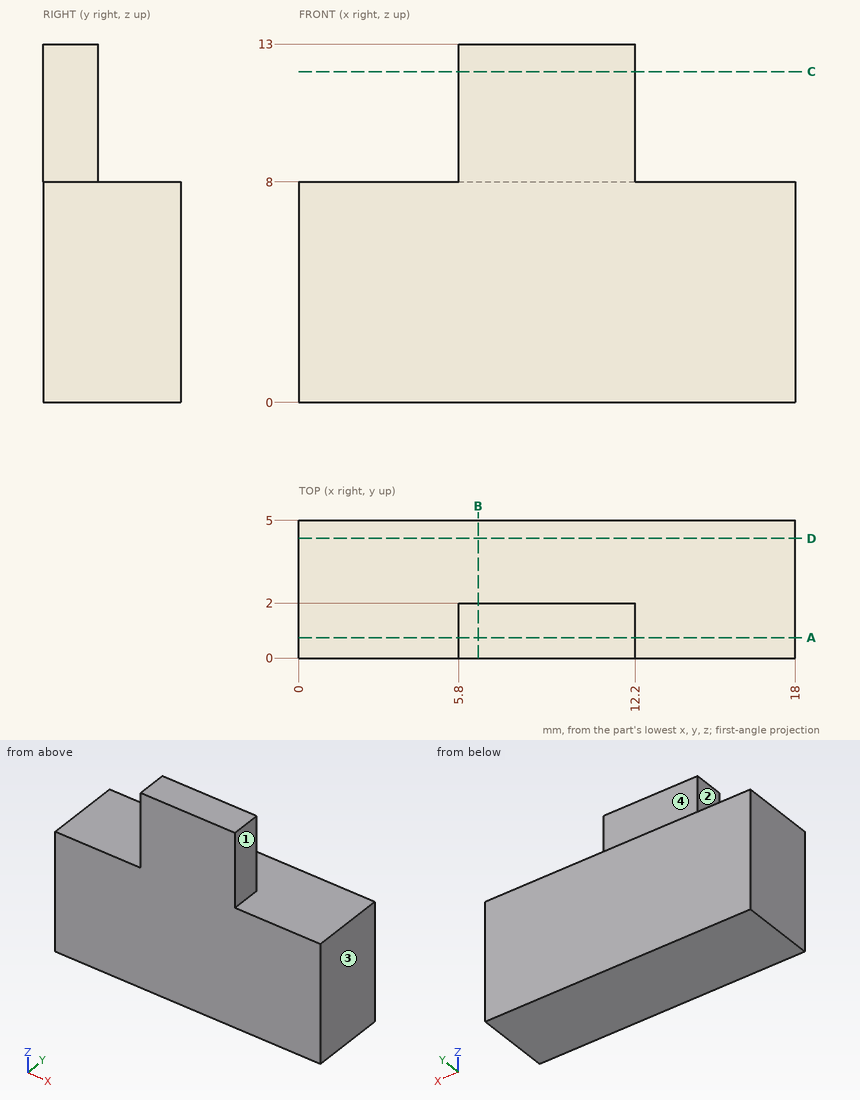
Verification items for this drawing (mm, ordinates from the low corner). A direction names the side the tool comes from. Coordinates: 2 decimals unless noted, no trailing zeros. Loops run counter-clockwise (first coordinate to the right, second up) from the corner with the lowest first, then second, coordinate; pieces in that order, holes last. Notation, with made-up numbers: (72, -22) -> (120, -22) arc R19 cw to (120, 13) -> close; hole circle Ø8 at (54, -9.5). An arc over 180 degrees is marked (long way). Answer in a Markdown table with one row per item. Add a question column.
1. Section check D-D, the plane y = 4.35. Enter the section's corners in (x, z).
2. Section check A-A, the plane y = 0.75. Enter the section's corners in (x, z), then the cut area to 3 significant figures.
3. Section check B-B, the plane x = 6.5. Enter the section's corners in (y, z), then the cut area to 3 significant figures.
4. Section check C-C, the plane z = 12. Enter the section's corners in (x, y).
5. Material ranges on probe 1 along Z at (x, y) = (0.5, 4.2); probe 2 along X at (y, z) = (0.7, 10.5); probe 3 along Y at (x, z) = (6, 10.5), recorded low to high. Write a range as [from, to].
6. Access from +Z, -Z, +X, -X, +Y, -Y to the whole of each face (thin tool, end or side, straight path). Record for the marked faces 1, 2, 3 and 4.
7. Depth check by flat-ended pin: P1, Ø1, axis at y = 1, z = 10, coming from the -X side; P2, Ø1, axis at y = 1, z = 9.5, coming from the +X side; P3, Ø1, axis at x = 12, z = 11, coming from the +Y side. Enter the tip coordinate at first touch or a pass-through.
Derived:
| question | item | result |
|---|---|---|
| 1 | outline | (0, 0) -> (18, 0) -> (18, 8) -> (0, 8) -> close |
| 2 | outline | (0, 0) -> (18, 0) -> (18, 8) -> (12.2, 8) -> (12.2, 13) -> (5.8, 13) -> (5.8, 8) -> (0, 8) -> close |
| 2 | area | 176 mm² |
| 3 | outline | (0, 0) -> (5, 0) -> (5, 8) -> (2, 8) -> (2, 13) -> (0, 13) -> close |
| 3 | area | 50.0 mm² |
| 4 | outline | (5.8, 0) -> (12.2, 0) -> (12.2, 2) -> (5.8, 2) -> close |
| 5 | probe 1 | z = [0, 8] |
| 5 | probe 2 | x = [5.8, 12.2] |
| 5 | probe 3 | y = [0, 2] |
| 6 | face 1 | +Z, +X, +Y, -Y |
| 6 | face 2 | +Z, -X, +Y, -Y |
| 6 | face 3 | +Z, -Z, +X, +Y, -Y |
| 6 | face 4 | +Z, +X, -X, +Y |
| 7 | P1 | stops at x = 5.8 |
| 7 | P2 | stops at x = 12.2 |
| 7 | P3 | stops at y = 2 |
